Verification items for the finished model (mm, model axes). A direction names the side the tool comes from. Give positions to 0.01 mm unless a question says otherwise; leave off trailing zeros. Order: outer loops, then holes, each group sorted by start corner. A loop starts at its lowest first (then second) coordinate and runs counter-clockwise, first axis right, second up. Notation, with made-up numbers: (21, -35) -> (57, -35) arc R15 ccw to (57, -9) -> close; hole circle Ø5 at (-17.75, 88.25). An arc over 180 degrees is marked (long way). Return JSON: item names as keys, results as strings. Group by question number.
(1) Cross-section at C-C on y = -13.5. Enter the section's corners in (x, z).
(2) Release check for a two-part mould opening along X. For faces 1 (the face through (-0.83, -7.26, 6.31)), 2 (the face through (-7, -14.732, 0)), 3 (the face through (-7.559, -0.859, -5.796)) record: pulls with the +X half, pulls with the -X half, needs draft (parallel to the pull), parting line crosses it, or undercut.
(3) Cross-section at A-A on z = 0. Enter the section's corners in (x, y) (3 decimals), then the cut area to 3 significant figures.
(4) Depth check by flat-ended pin: pin 1 Ø6 at (y, z) = (-9.5, 3) entering from +X; pin 2 Ø8 at (x, y) = (-2, -6) entering from -Z; pin 3 Ø1.5 at (x, y) = (-0.5, -2) entering from +Z. Enter the tip coordinate at first touch or a pass-through.
(5) Tool access check on faces 4 (the face through (4, 0, -6)), 5 (the face through (-4, -1.219, 7)). Record the directions out of +Z, -Z, +X, -X, +Y, -Y that give a thin tool (end or side, any length) a straight path to the whole face; none if there is none.
(6) Thickness scan on line 1 along Z through (x, y) = (0, -11); line 2 along Y through (x, z) = (-4, -7.75); line 3 along X through (y, z) = (-6, 4). Record the ranges inside material, lowest first.
(7) Cross-section at B-B on x = 0. Enter the section's corners in (y, z) (3 decimals).
from build123d import *

# Parameters (mm, degrees)
F0_R     = 9.525
F0_R_2   = 6.3627
F1_DEPTH = 1.2192
F2_R     = 7.88035
F2_R_2   = 6.3627
F3_DEPTH = 13.5128
F4_SIZE2 = 0.508
F4_SIZE  = 0.508


with BuildPart() as f1:
    # F0 (on Front) → F1 (new body)
    with BuildSketch(Plane.XZ):
        Circle(F0_R)
        Circle(F0_R_2, mode=Mode.SUBTRACT)
    extrude(amount=F1_DEPTH)

    # F2 (on face) → F3 (join)
    with BuildSketch(Plane.XZ.offset(1.2192)):
        Circle(F2_R)
        Circle(F2_R_2, mode=Mode.SUBTRACT)
    extrude(amount=F3_DEPTH)

    # F4
    f4_edges = [f1.edges().sort_by_distance(p)[0] for p in [
        (-9.525, 0, 0),
        (-7.88035, -14.732, 0),
    ]]
    chamfer(f4_edges, length=F4_SIZE, length2=F4_SIZE2)


solid = f1.part
Verdict:
{
 "1": {"outline": "circle Ø15.76 at (0, 0); hole circle Ø12.73 at (0, 0)"},
 "2": {"face 1": "undercut", "face 2": "needs draft", "face 3": "parting line crosses it"},
 "3": {"outline": "(-9.525, -1.219) -> (-7.88, -1.219) -> (-7.88, -14.224) -> (-7.372, -14.732) -> (-6.363, -14.732) -> (-6.363, 0) -> (-9.017, 0) -> (-9.525, -0.508) -> close; (6.363, -14.732) -> (7.372, -14.732) -> (7.88, -14.224) -> (7.88, -1.219) -> (9.525, -1.219) -> (9.525, -0.508) -> (9.017, 0) -> (6.363, 0) -> close", "area": "48.2 mm²"},
 "4": {"pin 1": "x = 7.88", "pin 2": "z = -7.88", "pin 3": "z = 7.88"},
 "5": {"face 4": "+Z, -Z, +X, -X, +Y", "face 5": "-Y"},
 "6": {"line 1": "-7.88 to -6.36, 6.36 to 7.88", "line 2": "-1.22 to 0", "line 3": "-6.79 to -4.95, 4.95 to 6.79"},
 "7": {"outline": "(-14.732, -7.372) -> (-14.224, -7.88) -> (-1.219, -7.88) -> (-1.219, -9.525) -> (-0.508, -9.525) -> (0, -9.017) -> (0, -6.363) -> (-14.732, -6.363) -> close; (-14.732, 6.363) -> (0, 6.363) -> (0, 9.017) -> (-0.508, 9.525) -> (-1.219, 9.525) -> (-1.219, 7.88) -> (-14.224, 7.88) -> (-14.732, 7.372) -> close"}
}
